```python
from build123d import *

# Parameters (mm, degrees)
SKETCH1_W           = 1092.2
SKETCH1_H           = 1168.4
BOSS_EXTRUDE1_DEPTH = 12.7
SKETCH2_W           = 1092.2
SKETCH2_H           = 1168.4
SKETCH2_W_2         = 1066.8
SKETCH2_H_2         = 1143
BOSS_EXTRUDE2_DEPTH = 215.9
SKETCH3_W           = 38.1
SKETCH3_H           = 38.1
BOSS_EXTRUDE3_DEPTH = 1168.4


with BuildPart() as part:
    # Sketch1 → Boss-Extrude1 (new body)
    with BuildSketch(Plane(origin=(0, 0, 0), x_dir=(1, 0, 0), z_dir=(0, 1, 0))):
        Rectangle(SKETCH1_W, SKETCH1_H)
    extrude(amount=BOSS_EXTRUDE1_DEPTH)

    # Sketch2 → Boss-Extrude2 (add)
    with BuildSketch(Plane(origin=(0, 12.7, 0), x_dir=(1, 0, 0), z_dir=(0, 1, 0))):
        Rectangle(SKETCH2_W, SKETCH2_H)
        Rectangle(SKETCH2_W_2, SKETCH2_H_2, mode=Mode.SUBTRACT)
    extrude(amount=BOSS_EXTRUDE2_DEPTH)

    # Sketch3 → Boss-Extrude3 (add)
    with BuildSketch(Plane(origin=(0, 0, -584.2), x_dir=(-1, 0, 0), z_dir=(0, 0, -1))):
        with Locations((565.15, 69.85)):
            Rectangle(SKETCH3_W, SKETCH3_H)
        with Locations((-565.15, 69.85)):
            Rectangle(SKETCH3_W, SKETCH3_H)
    extrude(amount=-BOSS_EXTRUDE3_DEPTH)


solid = part.part
```
Can you work these out from the model? Positions are in its coordinate system, mm. A direction names the side the tool comes from. Round coordinates to 2 decimals unless told otherwise and drop trailing zeros. Loops run counter-clockwise (first coordinate to the right, second up) from the corner with the lowest first, then second, coordinate; pieces in that order, holes last. Notation, with made-up numbers: M 16,1.5 L 34,1.5 A26 ccw 34,39.5 Z; hole C 67.5,39.25 d5. An arc over 180 degrees is marked long. Answer as a JSON object with one key per item and string values. Group by question number.
Q1. We'd pull the mould along X, two halves only. Please class faces 6 (the flat face through (-7, 12.7, -8)), 7 (the flat face through (-584.2, 70, -8)), 8 (the flat face through (-7, 119, 571.5)), 9 (the flat face through (-565, 50.8, -8)): +X half, -X half, draft (parallel to the pull), parting line (faces both ways), or undercut.
Q2. Will these pins go through, and if not, where does the flat tip stop? pin 1 (11.5 mm diameter, centred on x = -570, z = -231, fed in from +Y); pin 2 (11.5 mm diameter, centred on x = 559.5, z = -213, fed in from -Y); pin 3 (12 mm diameter, centred on y = 137.5, z = 17.5, fed in from -X).
Q3. Please list where these lines run through material, in increasing order: L1, parallel to Z at x = 406, y = 14.5; L2, parallel to X at y = 97.5, z = 355; L3, parallel to X at y = 71, z = 364.
Q4. Imagine slicing it at A-A, the plane y = 159. Please give me the cut outline in (x, z).
Q5. On a 3-axis mill with a long thin cutter (end or side, diameter ignored), from which of +Z, -Z, +X, -X, +Y, -Y can I reach the whole of each face in a straight line? I mean faces 1 (the flat face through (-533.4, 119, 8)), 2 (the flat face through (565, 88.9, -8)), 3 (the flat face through (546.1, 25, 8)), 4 (the flat face through (-546.1, 158, 8)), 5 (the flat face through (-546.1, 25, 8)). Say none if no direction works.
Q6. Imagine slicing it at B-B, the plane x = 78. Please give me the cut outline in (y, z), then the cut area to 3 significant figures.
Q7. Imagine slicing it at C-C, the plane z = -348. Please give me the cut outline in (x, y), then the cut area to 3 significant figures.
Findings:
{
 "1": {"face 6": "undercut", "face 7": "-X half", "face 8": "undercut", "face 9": "draft"},
 "2": {"pin 1": "stops at y = 88.9", "pin 2": "stops at y = 50.8", "pin 3": "stops at x = -546.1"},
 "3": {"L1": "z = -584.2 to -571.5, 571.5 to 584.2", "L2": "x = -546.1 to -533.4, 533.4 to 546.1", "L3": "x = -584.2 to -533.4, 533.4 to 584.2"},
 "4": {"outline": "M -546.1,-584.2 L 546.1,-584.2 L 546.1,584.2 L -546.1,584.2 Z; hole M -533.4,-571.5 L 533.4,-571.5 L 533.4,571.5 L -533.4,571.5 Z"},
 "5": {"face 1": "+Y", "face 2": "+Z, -Z, +X, +Y", "face 3": "+Z, -Z, +X, -Y", "face 4": "+Z, -Z, -X, +Y", "face 5": "+Z, -Z, -X, -Y"},
 "6": {"outline": "M 0,-584.2 L 228.6,-584.2 L 228.6,-571.5 L 12.7,-571.5 L 12.7,571.5 L 228.6,571.5 L 228.6,584.2 L 0,584.2 Z", "area": "20,300 mm2"},
 "7": {"outline": "M -584.2,50.8 L -546.1,50.8 L -546.1,0 L 546.1,0 L 546.1,50.8 L 584.2,50.8 L 584.2,88.9 L 546.1,88.9 L 546.1,228.6 L 533.4,228.6 L 533.4,12.7 L -533.4,12.7 L -533.4,228.6 L -546.1,228.6 L -546.1,88.9 L -584.2,88.9 Z", "area": "22,300 mm2"}
}
